Input: part model. Units: mm. Frame: model coordinates. Coordinates: 2 decimals unless noted, no trailing zeros. Write each loop counter-clockwise with the first axis right and the second up, starting at its lowest first coordinate (ties: lowest second). Pieces come first, ordered by that corner, then holes. Notation, with made-up numbers: (16, 17) - (62, 17) arc R11 ccw to (62, 34) - close; hole circle Ø2 at (-23, 52). An arc over 180 degrees is marked (long way). Use a Markdown table: item, result. Add a question column.
Q1. Section query C-C (z = -14.25). Return the cut outline in (x, y), then the cut area to 3 significant figures.
Q2. Section query B-B (y = 2.3). Return the cut outline in (x, z), then the cut area to 3 significant figures.
Q3. Section query A-A (x = 14). Return the cut outline in (y, z), then the cut area to 3 significant figures.
Q4. Material intervals for probe 1 along Z at (x, y) = (-7, 1.95); probe 2 along X at (y, z) = (1.1, -14.25); probe 3 along Z at (x, y) = (18, 2.1), sorted ascending. Write a range as from..to.
from build123d import *

# Parameters (mm, degrees)
SKETCH1_W           = 68.4
SKETCH1_H           = 45.8
BOSS_EXTRUDE1_DEPTH = 3
SKETCH2_R           = 0.95
CUT_EXTRUDE1_DEPTH  = 42.268026364
SKETCH3_W           = 23
SKETCH3_H           = 6
SKETCH3_W_2         = 46
SKETCH3_H_2         = 6.5
CUT_EXTRUDE2_DEPTH  = 42.268026364


with BuildPart() as part:
    # Sketch1 → Boss-Extrude1 (new body)
    with BuildSketch(Plane(origin=(0, 0, 0), x_dir=(1, 0, 0), z_dir=(0, 1, 0))):
        Rectangle(SKETCH1_W, SKETCH1_H)
    extrude(amount=BOSS_EXTRUDE1_DEPTH)

    # Sketch2 → Cut-Extrude1 (cut, through all)
    with BuildSketch(Plane(origin=(0, 3, 0), x_dir=(1, 0, 0), z_dir=(0, 1, 0))):
        with Locations(Location((-20.32, 14.25, 0), (0, 0, 270))):
            Circle(SKETCH2_R)
        with Locations(Location((20.32, 14.25, 0), (0, 0, 90))):
            Circle(SKETCH2_R)
    extrude(amount=-CUT_EXTRUDE1_DEPTH, mode=Mode.SUBTRACT)

    # Sketch3 → Cut-Extrude2 (cut, through all)
    with BuildSketch(Plane(origin=(0, 3, 0), x_dir=(1, 0, 0), z_dir=(0, 1, 0))):
        with Locations((0, 13.9)):
            Rectangle(SKETCH3_W, SKETCH3_H)
        with Locations((0, -8.35)):
            Rectangle(SKETCH3_W_2, SKETCH3_H_2)
    extrude(amount=-CUT_EXTRUDE2_DEPTH, mode=Mode.SUBTRACT)


solid = part.part
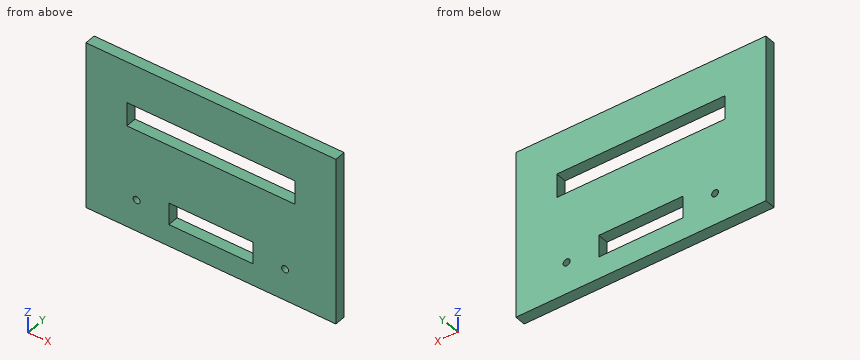
Values follow:
| question | item | result |
|---|---|---|
| 1 | outline | (-34.2, 0) - (-21.27, 0) - (-21.27, 3) - (-34.2, 3) - close; (-19.37, 0) - (-11.5, 0) - (-11.5, 3) - (-19.37, 3) - close; (11.5, 0) - (19.37, 0) - (19.37, 3) - (11.5, 3) - close; (21.27, 0) - (34.2, 0) - (34.2, 3) - (21.27, 3) - close |
| 1 | area | 125 mm2 |
| 2 | outline | (-34.2, -22.9) - (34.2, -22.9) - (34.2, 22.9) - (-34.2, 22.9) - close; hole (-23, 5.1) - (23, 5.1) - (23, 11.6) - (-23, 11.6) - close; hole circle Ø1.9 at (-20.32, -14.25); hole (-11.5, -16.9) - (11.5, -16.9) - (11.5, -10.9) - (-11.5, -10.9) - close; hole circle Ø1.9 at (20.32, -14.25) |
| 2 | area | 2,690 mm2 |
| 3 | outline | (0, -22.9) - (3, -22.9) - (3, 5.1) - (0, 5.1) - close; (0, 11.6) - (3, 11.6) - (3, 22.9) - (0, 22.9) - close |
| 3 | area | 118 mm2 |
| 4 | probe 1 | -22.9..-16.9, -10.9..5.1, 11.6..22.9 |
| 4 | probe 2 | -34.2..-21.27, -19.37..-11.5, 11.5..19.37, 21.27..34.2 |
| 4 | probe 3 | -22.9..5.1, 11.6..22.9 |
